Read the model definition and answer for the solid it produces. Units are mm, in the model's axes. A direction names the side the tool comes from. Coordinates: 2 decimals unless noted, no trailing zeros. Order: outer loops, then holes, each group sorted by start corner. A loop starts at its lowest first (then second) coordinate and runs counter-clockwise, first axis right, second up.
Autodesk Inventor part; units mm, degrees
ref_plane "YZ Plane" through (0, 0, 0) normal (1, 0, 0) x (0, 1, 0)
ref_plane "XZ Plane" through (0, 0, 0) normal (0, 1, 0) x (-1, 0, 0)
ref_plane "XY Plane" through (0, 0, 0) normal (0, 0, 1) x (1, 0, 0)
sketch "スケッチ1" plane through (0, 0, 0) normal (0, 1, 0) x (-1, 0, 0)
  line L0 (3, 0) -> (6, 0)
  line L1 (6, 0) -> (6, 1.5)
  line L2 (6, 1.5) -> (5, 1.5)
  line L3 (5, 1.5) -> (5, 5)
  line L4 (4.5, 6) -> (3, 6)
  line L5 (3, 6) -> (3, 0)
  line L6 (5, 5) -> (4.5, 6)
  line L7 (0, -1.2) -> (0, 7.2)
  point P0 (0, 0)
  point P1 (3, 6)
  dimension "d5" = 1.5
  dimension "d9" = 1
  dimension "d10" = 0.5
  dimension "d17" = 10
  dimension "d18" = 12
  dimension "d19" = 6
  dimension "d20" = 6
revolve "回転1" add sketch "スケッチ1" angle 360 about axis through (0, 0, -10) along (0, 0, 1)
sketch "スケッチ2" plane through (0, 0, 6) normal (0, 0, 1) x (1, 0, 0)
  line L0 (4.4, -2.3749) -> (-4.4, -2.3749)
  line L1 (-4.4, -2.3749) -> (-4.4, 2.3749)
  line L2 (-4.4, 2.3749) -> (4.4, 2.3749)
  line L3 (4.4, 2.3749) -> (4.4, -2.3749)
  line L4 (4.4, -2.3749) -> (-4.4, 2.3749) construction
  line L5 (-4.4, -2.3749) -> (4.4, 2.3749) construction
  circle A0 centre (0, 0) radius 5
  point P0 (0, 0)
  dimension "d12" = 10
  dimension "d11" = 8.8
extrude "押し出し1" cut sketch "スケッチ2" against normal up to surface (4.5 mm away) contours L3 A0 | A0 L1
properties part number "LED-0606" material "アセタール樹脂、黒"
1) A cutting plane is placed at D-D, the plane z = 4. Determine the outline of the cut face in (x, y).
A:
outline: (-4.4, -2.37) arc R5 ccw to (4.4, -2.37) - (4.4, 2.37) arc R5 ccw to (-4.4, 2.37) - close; hole circle Ø6 at (0, 0)
2) Which of the six approach directions +Z, -Z, +X, -X, +Y, -Y give full straight-line access (tool end or side, diameter ignored) to faces 4 (the cylindrical face through (6, 0, 1)), 5 (the flat face through (4.4, 0, 4)), 6 (the cylindrical face through (0, 5, 3)), 7 (the flat face through (-4.4, 0, 4))?
A:
face 4: +Z, -Z
face 5: +Z, +X, +Y, -Y
face 6: +Z, +Y
face 7: +Z, -X, +Y, -Y
3) Determine the mould class of faces 1 (the cylindrical face through (3, 0, 3)), 2 (the flat face through (3, 1, 0)), 3 (the cylindrical face through (0, -5, 3)) for opening direction X: pulls with the +X half, pulls with the -X half, needs draft (parallel to the pull), parting line crosses it, or undercut.
A:
face 1: undercut
face 2: needs draft
face 3: parting line crosses it
4) Flat-ended cylindrical pins translate along their axes: pin 1 Ø3.5 at (y, z) = (-0.5, 4.5) entering from -X; pin 2 Ø1.4 at (y, z) = (0, 3.5) entering from +X. Find the tip coordinate at first contact, or state that the pin passes through.
A:
pin 1: stops at x = -4.4
pin 2: stops at x = 4.4
5) A cutting plane is placed at A-A, the plane x = 0. Determine the outline of the cut face in (y, z), and give its area (3 significant figures).
A:
outline: (-6, 0) - (-3, 0) - (-3, 6) - (-4.5, 6) - (-5, 5) - (-5, 1.5) - (-6, 1.5) - close; (3, 0) - (6, 0) - (6, 1.5) - (5, 1.5) - (5, 5) - (4.5, 6) - (3, 6) - close
area: 26.5 mm2
6) A cutting plane is placed at C-C, the plane z = 5.75. Determine the outline of the cut face in (x, y) (3 decimals), and give its area (3 significant figures).
A:
outline: (-4.4, -1.425) arc R4.625 ccw to (4.4, -1.425) - (4.4, 1.425) arc R4.625 ccw to (-4.4, 1.425) - close; hole circle Ø6 at (0, 0)
area: 38.1 mm2
7) Straight lines are drawn through the part: line 1 (X direction, y = 0, z = 3.9); line 2 (Y direction, x = 2.25, z = 2); line 3 (Y direction, x = 2, z = 5.25). For each, find the intervals that lie inside material, in ascending order.
A:
line 1: x = -4.4 to -3, 3 to 4.4
line 2: y = -4.47 to -1.98, 1.98 to 4.47
line 3: y = -4.45 to -2.24, 2.24 to 4.45
8) A cutting plane is placed at B-B, the plane y = 0. Determine the outline of the cut face in (x, z).
A:
outline: (-6, 0) - (-3, 0) - (-3, 6) - (-4.4, 6) - (-4.4, 1.5) - (-6, 1.5) - close; (3, 0) - (6, 0) - (6, 1.5) - (4.4, 1.5) - (4.4, 6) - (3, 6) - close
